Source: three-view drawing plus pictorial views. Frame: mm from the lowest corner of the part. Round coordinates to 2 decimals unless told otherwise and drop trailing zeros. Write each loop counter-clockwise with the first axis right and the second up, starting at its lowest first coordinate (ties: lowest second). Pieces come first, ordered by that corner, then holes. Notation, with made-up numbers: (44.5, 6) - (61.5, 6) arc R31 cw to (61.5, 45) - close; hole circle Ø6 at (2.25, 62.5). An arc over 180 degrees is marked (long way). Write each question's results on one line, items separated by ' | '.
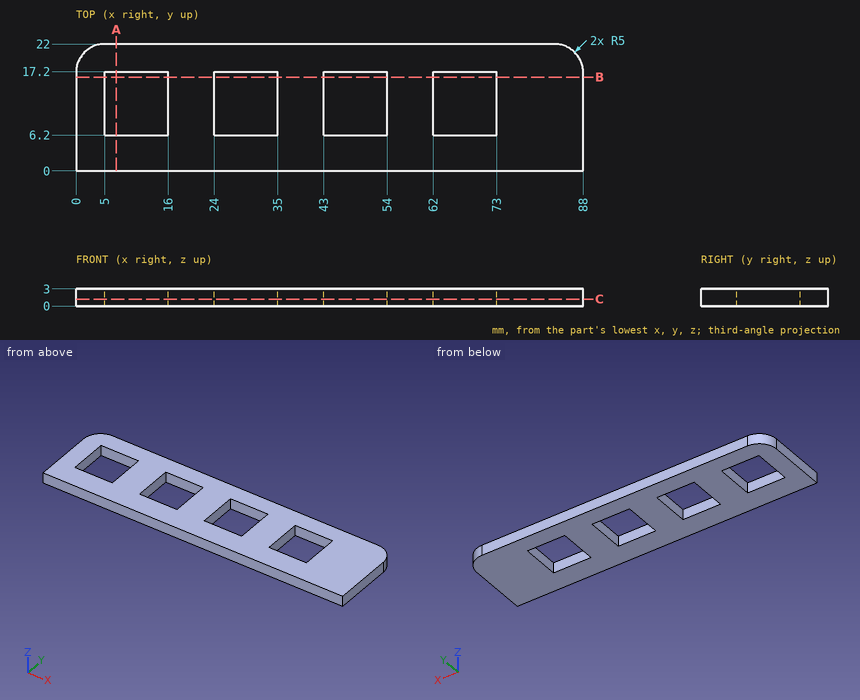
Q1. Section query C-C, the plane z = 1.2. Return loops of the section in (x, y), plus the area to 3 significant figures.
Answer block:
outline: (0, 0) - (88, 0) - (88, 17) arc R5 ccw to (83, 22) - (5, 22) arc R5 ccw to (0, 17) - close; hole (5, 6.2) - (16, 6.2) - (16, 17.2) - (5, 17.2) - close; hole (24, 6.2) - (35, 6.2) - (35, 17.2) - (24, 17.2) - close; hole (43, 6.2) - (54, 6.2) - (54, 17.2) - (43, 17.2) - close; hole (62, 6.2) - (73, 6.2) - (73, 17.2) - (62, 17.2) - close | area: 1,440 mm2
Q2. Section query A-A, the plane x = 7. Return loops of the section in (y, z).
Answer block:
outline: (0, 0) - (6.2, 0) - (6.2, 3) - (0, 3) - close; (17.2, 0) - (22, 0) - (22, 3) - (17.2, 3) - close
Q3. Pin query (flat end, axial travel): pin 1 (4 mm diameter, centred on x = 51, y = 13, fed in from -Z). Return the tip coordinate at first contact, or that it passes through.
Answer block:
pin 1: through
Q4. Ray query, line 1 along X through (y, z) = (14.75, 0.8); line 2 along Y through (x, z) = (46.5, 1.4); line 3 along X through (y, z) = (20, 0.8). Return the intervals inside material, ascending.
Answer block:
line 1: 0 to 5, 16 to 24, 35 to 43, 54 to 62, 73 to 88 | line 2: 0 to 6.2, 17.2 to 22 | line 3: 1 to 87
Q5. Section query B-B, the plane y = 16.25. Return loops of the section in (x, z).
Answer block:
outline: (0, 0) - (5, 0) - (5, 3) - (0, 3) - close; (16, 0) - (24, 0) - (24, 3) - (16, 3) - close; (35, 0) - (43, 0) - (43, 3) - (35, 3) - close; (54, 0) - (62, 0) - (62, 3) - (54, 3) - close; (73, 0) - (88, 0) - (88, 3) - (73, 3) - close
